from build123d import *

# Parameters (mm, degrees)
SKETCH004_R     = 1.475
PAD003_DEPTH    = 10
SKETCH009_R     = 2.76
POCKET002_DEPTH = 3
SKETCH014_R     = 11.1
POCKET006_DEPTH = 2
SKETCH042_R     = 11.1
POCKET026_DEPTH = 2


with BuildPart() as part:
    # Sketch004 → Pad003 (new body)
    with BuildSketch(Plane.XY):
        with BuildLine():
            Line((-21, 21), (21, 21))
            Line((21, 21), (21, 10))
            Line((21, 10), (0, 10))
            ThreePointArc((0, 10), (-10, 0), (0, -10))
            Line((21, -10), (0, -10))
            Line((21, -21), (21, -10))
            Line((21, -21), (-21, -21))
            Line((-21, -21), (-21, 21))
        make_face()
        with Locations((-15.5, 15.5)):
            Circle(SKETCH004_R, mode=Mode.SUBTRACT)
        with Locations((15.5, 15.5)):
            Circle(SKETCH004_R, mode=Mode.SUBTRACT)
        with Locations((-15.5, -15.5)):
            Circle(SKETCH004_R, mode=Mode.SUBTRACT)
        with Locations((15.5, -15.5)):
            Circle(SKETCH004_R, mode=Mode.SUBTRACT)
        with Locations((-15.5, 0)):
            Circle(SKETCH004_R, mode=Mode.SUBTRACT)
        with Locations((0, 15.5)):
            Circle(SKETCH004_R, mode=Mode.SUBTRACT)
        with Locations((0, -15.5)):
            Circle(SKETCH004_R, mode=Mode.SUBTRACT)
    extrude(amount=PAD003_DEPTH)

    # Sketch009 → Pocket002 (cut)
    with BuildSketch(Plane.XY):
        with Locations((-15.5, 15.5)):
            Circle(SKETCH009_R)
        with Locations((15.5, 15.5)):
            Circle(SKETCH009_R)
        with Locations((-15.5, -15.5)):
            Circle(SKETCH009_R)
        with Locations((15.5, -15.5)):
            Circle(SKETCH009_R)
        with Locations((-15.5, 0)):
            Circle(SKETCH009_R)
        with Locations((0, 15.5)):
            Circle(SKETCH009_R)
        with Locations((0, -15.5)):
            Circle(SKETCH009_R)
    extrude(amount=POCKET002_DEPTH, mode=Mode.SUBTRACT)

    # Sketch014 (on Face5 of Pocket002) → Pocket006 (cut)
    with BuildSketch(Plane.XY.offset(10)):
        Circle(SKETCH014_R)
    extrude(amount=-POCKET006_DEPTH, mode=Mode.SUBTRACT)

    # Sketch042 → Pocket026 (cut)
    with BuildSketch(Plane.XY):
        Circle(SKETCH042_R)
    extrude(amount=POCKET026_DEPTH, mode=Mode.SUBTRACT)


with BuildPart() as part_1:
    # Body003 placement: moved
    add(part.part.moved(Location((0, 0, -30))))


solid = part_1.part
Geometry check sheet. Reference: the model listing, model coordinates, mm. A direction names the side the tool comes from. Coordinates: 2 decimals unless noted, no trailing zeros. Loops run counter-clockwise (first coordinate to the right, second up) from the corner with the lowest first, then second, coordinate; pieces in that order, holes last. Notation, with made-up numbers: (43.25, 57) - (55.25, 57) arc R31 cw to (55.25, 91) - close; hole circle Ø10 at (31.25, -23.75). An arc over 180 degrees is marked (long way). Use one line per item in the form item = value. Start each with the question number.
Item 1: Section check A-A, the plane y = 15.5. Enter the section's corners in (x, z) (3 decimals).
Item 2: Tool access check on faces 1 (the face through (-14.093, 15.943, -23.549)), 2 (the face through (13.31, -17.18, -28.52)), 3 (the face through (-10.3, 0.1, -22)). Record the directions out of +Z, -Z, +X, -X, +Y, -Y that give a thin tool (end or side, any length) a straight path to the whole face; none if there is none.
Item 3: Thickness scan on probe 1 along Y at (x, z) = (-15.5, -28.45); probe 2 along X at (y, z) = (15.5, -24) (3 decimals); probe 3 along Y at (x, z) = (0, -29.2). Record the ranges inside material, lowest first.
Item 4: Section check C-C, the plane z = -25.75. Enter the section's corners in (x, y) (3 decimals).
Item 5: Gauge pin test, flat ends, axial feed: pin 1 (12 mm diameter, centred on x = 10, y = 3.5, fed in from +Z); pin 2 (5 mm diameter, centred on x = 15.5, y = 15.5, fed in from -Z); pin 3 (1 mm diameter, centred on y = -7, z = -24.5, fed in from +X). Record the tip position at first contact, or that the pin passes through.
Item 6: Mould release check, pull along X, two halves, no side actions. Record for faces 4 (the face through (11, 10, -25)), 5 (the face through (-10.3, 0.1, -28)), 6 (the face through (-0.359, 18.237, -28.521)), 7 (the face through (-21, 0, -25)): +X half, -X half, draft (parallel to the pull), parting line (faces both ways), or undercut.
Item 7: Section check D-D, the plane x = 9. Enter the section's corners in (y, z), and give its area (3 significant figures).
Item 8: Section check B-B, the plane x = 15.5. Enter the section's corners in (y, z) (3 decimals), and give its area (3 significant figures).
Computed:
q1.outline = (-21, -30) - (-18.26, -30) - (-18.26, -27) - (-16.975, -27) - (-16.975, -20) - (-21, -20) - close; (-14.025, -27) - (-12.74, -27) - (-12.74, -30) - (-2.76, -30) - (-2.76, -27) - (-1.475, -27) - (-1.475, -20) - (-14.025, -20) - close; (1.475, -27) - (2.76, -27) - (2.76, -30) - (12.74, -30) - (12.74, -27) - (14.025, -27) - (14.025, -20) - (1.475, -20) - close; (16.975, -27) - (18.26, -27) - (18.26, -30) - (21, -30) - (21, -20) - (16.975, -20) - close
q2.face_1 = +Z, -Z
q2.face_2 = -Z
q2.face_3 = +Z
q3.probe_1 = -21 to -18.26, -12.74 to -2.76, 2.76 to 12.74, 18.26 to 21
q3.probe_2 = -21 to -16.975, -14.025 to -1.475, 1.475 to 14.025, 16.975 to 21
q3.probe_3 = -21 to -18.26, -12.74 to -11.1, 11.1 to 12.74, 18.26 to 21
q4.outline = (-21, -21) - (21, -21) - (21, -10) - (0, -10) arc R10 cw to (0, 10) - (21, 10) - (21, 21) - (-21, 21) - close; hole circle Ø2.95 at (-15.5, -15.5); hole circle Ø2.95 at (-15.5, 0); hole circle Ø2.95 at (-15.5, 15.5); hole circle Ø2.95 at (0, -15.5); hole circle Ø2.95 at (0, 15.5); hole circle Ø2.95 at (15.5, -15.5); hole circle Ø2.95 at (15.5, 15.5)
q5.pin_1 = through
q5.pin_2 = -27
q5.pin_3 = -6.61
q6.face_4 = draft
q6.face_5 = undercut
q6.face_6 = undercut
q6.face_7 = -X half
q7.outline = (-21, -30) - (-10, -30) - (-10, -20) - (-21, -20) - close; (10, -30) - (21, -30) - (21, -20) - (10, -20) - close
q7.area = 220 mm2
q8.outline = (-21, -30) - (-18.26, -30) - (-18.26, -27) - (-16.975, -27) - (-16.975, -20) - (-21, -20) - close; (-14.025, -27) - (-12.74, -27) - (-12.74, -30) - (-10, -30) - (-10, -20) - (-14.025, -20) - close; (10, -30) - (12.74, -30) - (12.74, -27) - (14.025, -27) - (14.025, -20) - (10, -20) - close; (16.975, -27) - (18.26, -27) - (18.26, -30) - (21, -30) - (21, -20) - (16.975, -20) - close
q8.area = 146 mm2
